Could you check a few things on this model? Use its own coordinates, in mm. Coordinates: 2 decimals unless noted, no trailing zeros. Loops run counter-clockwise (first coordinate to the right, second up) from the corner with the lowest first, then second, coordinate; pieces in that order, holes last. Notation, with made-up numbers: (5, 88.5) - (40, 88.5) arc R19 cw to (40, 97.5) - close; hole circle Ø3 at (13, 19.5). An arc over 180 degrees is marked (long way). One line per item, written item: value. Start each with the question number.
(1) I'm going to push flat-ended pins straight in: P1, Ø1.8, axis at x = 46.5, y = 0, coming from the +Z side; P2, Ø3, axis at x = 21, z = 3.5, coming from the -Y side; P3, Ø2, axis at y = 21, z = 3.5, coming from the -X side. Where does each tip first touch, or does it pass through?
(2) If I drill on line 1 along Y through (x, z) = (-47.05, 0.65); line 2 along X through (y, z) = (-14, 2.25); line 3 along Z through (x, y) = (-4, 11), over which ranges is the centre line in solid material (lowest first)? Write a range as from..to.
(3) If we section it at A-A on y = 9: Write out the boundary of the cut face in (x, z).
(4) If we section it at D-D on z = 3: Write out the boundary of the cut face in (x, y).
```python
from build123d import *
from build123d.topology import SkipClean

# Parameters (mm, degrees)
BOSS_EXTRUDE1_DEPTH        = 1.54
F_3_2_3_2_DIAMETER_HOLE1_D = 3.2
SKETCH4_R                  = 2.25
SKETCH4_R_2                = 1.6
BOSS_EXTRUDE2_DEPTH        = 0.1
SKETCH5_W                  = 85.5
SKETCH5_H                  = 54.969341598
BOSS_EXTRUDE3_DEPTH        = 3.7
SKETCH6_W                  = 73.44
SKETCH6_H                  = 48.96
CUT_EXTRUDE1_DEPTH         = 0.05
SKETCH7_W                  = 6
SKETCH7_H                  = 15
BOSS_EXTRUDE4_DEPTH        = 7.1
SKETCH8_W                  = 4.418406876
SKETCH8_H                  = 12.715571876
CUT_EXTRUDE2_DEPTH         = 6
BOSS_EXTRUDE5_DEPTH        = 1.88


with BuildPart() as part:
    # Sketch1 → Boss-Extrude1 (new body)
    with BuildSketch(Plane.XY):
        with BuildLine():
            Line((-47.25, 27.5), (47.25, 27.5))
            ThreePointArc((47.25, 27.5), (49.371320344, 26.621320344), (50.25, 24.5))
            Line((50.25, 24.5), (50.25, -24.5))
            ThreePointArc((50.25, -24.5), (49.371320344, -26.621320344), (47.25, -27.5))
            Line((47.25, -27.5), (-47.25, -27.5))
            ThreePointArc((-47.25, -27.5), (-49.371320344, -26.621320344), (-50.25, -24.5))
            Line((-50.25, -24.5), (-50.25, 24.5))
            ThreePointArc((-50.25, 24.5), (-49.371320344, 26.621320344), (-47.25, 27.5))
        make_face()
    extrude(amount=BOSS_EXTRUDE1_DEPTH)

    # Ø3.2 (3.2) Diameter Hole1 (through all)
    with Locations(Plane.XY.offset(1.54)):
        with Locations((-47.05, 24.25), (47.05, 24.25), (47.05, -24.25), (-47.05, -24.25)):
            Hole(F_3_2_3_2_DIAMETER_HOLE1_D / 2)

    # Sketch4 → Boss-Extrude2 (add)
    # profile 1 of 4: a face of its own
    with SkipClean():  # the faces are left unmerged after this step: merging them gives an invalid solid
        with BuildSketch(Plane.XY.offset(1.54)):
            with Locations((-47.05, 24.25)):
                Circle(SKETCH4_R)
            with Locations((-47.05, 24.25)):
                Circle(SKETCH4_R_2, mode=Mode.SUBTRACT)
        # profile 2 of 4: a face of its own
        with BuildSketch(Plane.XY.offset(1.54)):
            with Locations((-47.05, -24.25)):
                Circle(SKETCH4_R)
            with Locations((-47.05, -24.25)):
                Circle(SKETCH4_R_2, mode=Mode.SUBTRACT)
        # profile 3 of 4: a face of its own
        with BuildSketch(Plane.XY.offset(1.54)):
            with Locations((47.05, -24.25)):
                Circle(SKETCH4_R)
            with Locations((47.05, -24.25)):
                Circle(SKETCH4_R_2, mode=Mode.SUBTRACT)
        # profile 4 of 4: a face of its own
        with BuildSketch(Plane.XY.offset(1.54)):
            with Locations((47.05, 24.25)):
                Circle(SKETCH4_R)
            with Locations((47.05, 24.25)):
                Circle(SKETCH4_R_2, mode=Mode.SUBTRACT)
        extrude(amount=BOSS_EXTRUDE2_DEPTH)
    add(part.part.scale(1), mode=Mode.REPLACE)  # the faces are merged on a copy

    # Sketch5 → Boss-Extrude3 (add)
    with BuildSketch(Plane.XY.offset(1.54)):
        Rectangle(SKETCH5_W, SKETCH5_H)
    extrude(amount=BOSS_EXTRUDE3_DEPTH)

    # Sketch6 → Cut-Extrude1 (cut)
    with BuildSketch(Plane.XY.offset(5.24)):
        with Locations((4.48, 0)):
            Rectangle(SKETCH6_W, SKETCH6_H)
    extrude(amount=-CUT_EXTRUDE1_DEPTH, mode=Mode.SUBTRACT)

    # Sketch7 → Boss-Extrude4 (add)
    with BuildSketch(Plane(origin=(50.25, 0, 0), x_dir=(0, 0, -1), z_dir=(1, 0, 0))):
        with Locations((3, 0)):
            Rectangle(SKETCH7_W, SKETCH7_H)
    extrude(amount=-BOSS_EXTRUDE4_DEPTH)

    # Sketch8 → Cut-Extrude2 (cut)
    with BuildSketch(Plane(origin=(50.25, 0, 0), x_dir=(0, 0, -1), z_dir=(1, 0, 0))):
        with Locations((2.548027157, 0)):
            Rectangle(SKETCH8_W, SKETCH8_H)
    extrude(amount=-CUT_EXTRUDE2_DEPTH, mode=Mode.SUBTRACT)

    # Sketch9 → Boss-Extrude5 (add)
    with BuildSketch(Plane(origin=(0, 0, 0), x_dir=(-1, 0, 0), z_dir=(0, 0, -1))):
        with BuildLine():
            Line((-30.25, 12.3), (-15.25, 12.3))
            Line((-15.25, 12.3), (-15.25, 26.9))
            Line((-15.25, 26.9), (-25.232632272, 26.9))
            ThreePointArc((-25.232632272, 26.9), (-25.480119645, 27.002512627), (-25.582632272, 27.25))
            Line((-25.582632272, 27.25), (-25.582632272, 27.3))
            Line((-25.582632272, 27.3), (-30.25, 27.3))
            Line((-30.25, 27.3), (-30.25, 12.3))
        make_face()
    extrude(amount=BOSS_EXTRUDE5_DEPTH)


solid = part.part
```
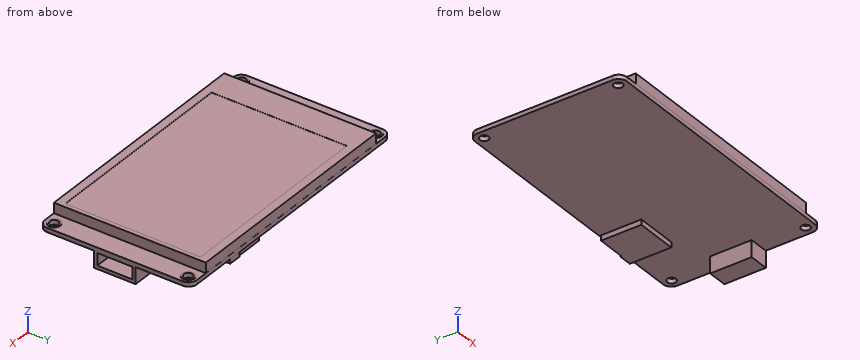
Values:
1. P1: stops at z = 1.54
1. P2: stops at y = -27.48
1. P3: stops at x = -42.75
2. line 1: y = -27.5..-25.85, -22.65..22.65, 25.85..27.5
2. line 2: x = -42.75..42.75
2. line 3: z = 0..5.19
3. outline: (-50.25, 0) - (50.25, 0) - (50.25, 1.54) - (42.75, 1.54) - (42.75, 5.24) - (41.2, 5.24) - (41.2, 5.19) - (-32.24, 5.19) - (-32.24, 5.24) - (-42.75, 5.24) - (-42.75, 1.54) - (-50.25, 1.54) - close
4. outline: (-42.75, -27.48) - (42.75, -27.48) - (42.75, 27.48) - (-42.75, 27.48) - close
